Here's how the part is built. I have some questions about the finished solid (model axes, mm). Round coordinates to 2 decimals unless told otherwise and drop trailing zeros. Order: outer loops, then holes, each group sorted by start corner. A loop starts at its lowest first (then second) coordinate and runs counter-clockwise, first axis right, second up. Notation, with made-up numbers: (30.25, 48.25) -> (48.25, 48.25) arc R14 ccw to (48.25, 57.25) -> close; hole circle Ø11 at (-37, 71). An arc over 180 degrees is marked (long way). Answer in a Markdown table with one row per item.
```python
from build123d import *

# Parameters (mm, degrees)
SKETCH1_W           = 76.2
SKETCH1_H           = 25.4
SKETCH1_R           = 3.175
BOSS_EXTRUDE1_DEPTH = 4.572


with BuildPart() as part:
    # Sketch1 → Boss-Extrude1 (new body)
    with BuildSketch(Plane.XY):
        Rectangle(SKETCH1_W, SKETCH1_H)
        with Locations((-28.575, 0)):
            Circle(SKETCH1_R, mode=Mode.SUBTRACT)
        with Locations((28.575, 0)):
            Circle(SKETCH1_R, mode=Mode.SUBTRACT)
    extrude(amount=-BOSS_EXTRUDE1_DEPTH)


solid = part.part
```
1. Suppose I cut it at C-C on x = -30. Write out the boundary of the cut face in (y, z), then the cut area to 3 significant figures.
Numbers:
| item | result |
|---|---|
| outline | (-12.7, -4.57) -> (-2.84, -4.57) -> (-2.84, 0) -> (-12.7, 0) -> close; (2.84, -4.57) -> (12.7, -4.57) -> (12.7, 0) -> (2.84, 0) -> close |
| area | 90.2 mm2 |
2. Suppose I cut it at A-A on y = 0. Write out the boundary of the cut face in (x, z).
Numbers:
| item | result |
|---|---|
| outline | (-38.1, -4.57) -> (-31.75, -4.57) -> (-31.75, 0) -> (-38.1, 0) -> close; (-25.4, -4.57) -> (25.4, -4.57) -> (25.4, 0) -> (-25.4, 0) -> close; (31.75, -4.57) -> (38.1, -4.57) -> (38.1, 0) -> (31.75, 0) -> close |
3. We'd pull the mould along X, two halves only. Please class faces 1 (the face through (25.4, 0.1, -2.3)), 2 (the face through (-31.095, -1.932, -2.254)), 3 (the face through (38.1, 0, -2)), 4 (the face through (-38.1, 0, -2)): released by +X, released by -X, zero draft, split by the parting line, or undercut.
Numbers:
| item | result |
|---|---|
| face 1 | undercut |
| face 2 | undercut |
| face 3 | released by +X |
| face 4 | released by -X |
4. Suppose I cut it at B-B on z = -1.35. Write out the boundary of the cut face in (x, y) (3 decimals), then the cut area to 3 significant figures.
Numbers:
| item | result |
|---|---|
| outline | (-38.1, -12.7) -> (38.1, -12.7) -> (38.1, 12.7) -> (-38.1, 12.7) -> close; hole circle Ø6.35 at (-28.575, 0); hole circle Ø6.35 at (28.575, 0) |
| area | 1,870 mm2 |
5. Please list where this line runs through material, in increasing order: line 1 along Y through (x, z) = (-26, -2.15).
Numbers:
| item | result |
|---|---|
| line 1 | y = -12.7 to -1.86, 1.86 to 12.7 |
